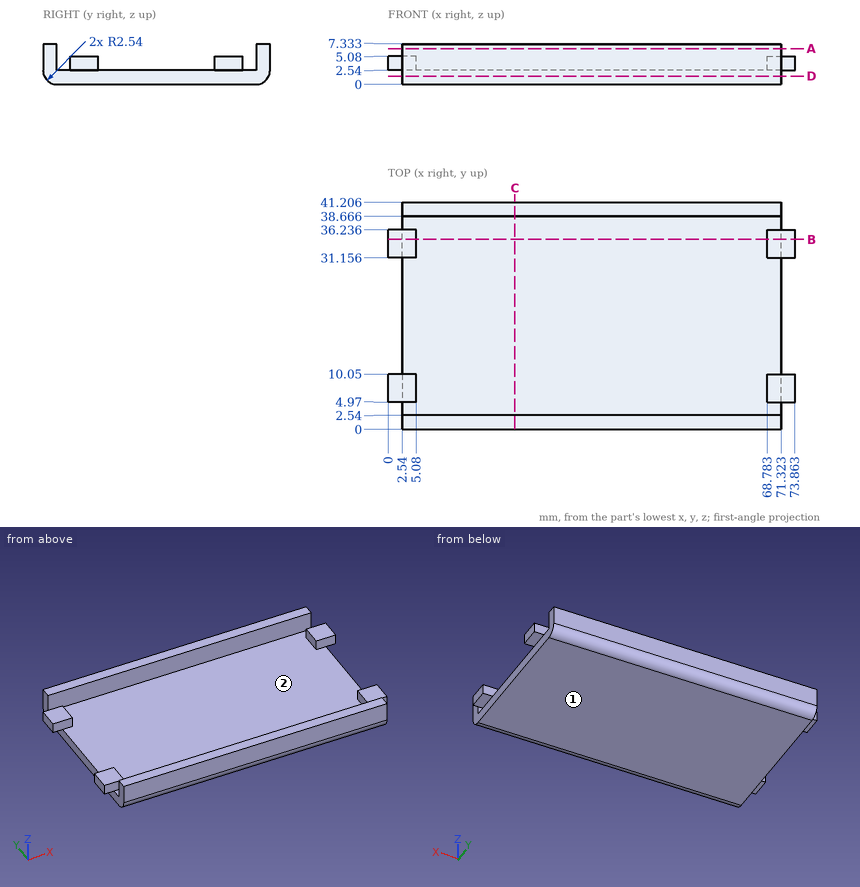
Answer from the drawing. Dimensions are ordinates in mm from the lowest x, y and z of the part. Give positions to 0.01 mm unless a question says otherwise; leave off trailing zeros. Write each loop counter-clockwise with the first axis right and the second up, starting at its lowest first coordinate (ties: lowest second). Pieces come first, ordered by that corner, then holes.
1) Find the intervals of material crossed by L1, parallel to X at y = 9, z = 2.75; L2, parallel to Y at x = 61, z = 6.75; L3, parallel to X at y = 16, z = 0.5, in increasing order.
2) Section C-C (x = 23) is taken. Write down the section's boundary in (y, z), and give its area (3 significant figures).
3) Section A-A (z = 6.5) is taken. Write down the section's boundary in (x, y).
4) For a pull along X with two mould halves and no side action, classify the marked faces 1 and 2 as pulls with the +X half, pulls with the -X half, needs draft (parallel to the pull), parting line crosses it, or undercut.
5) Given P1, Ø2, axis at y = 17, z = 4.5, coming from the +X side; P2, Ø1.3, axis at y = 34, z = 4, coming from the -X side; P3, Ø5.5, axis at x = 3, y = 34, coming from the +Z side; P4, Ø0.8, axis at x = 1.5, z = 4, coming from the +Y side, each flat-ended and moving along its own axis, determine where each tip first touches the part or whether it passes through.
6) Section B-B (y = 34.5) is taken. Write down the section's boundary in (x, z).
7) Section D-D (z = 1.5) is taken. Write down the section's boundary in (x, y).
Response:
1. L1: x = 0 to 5.08, 68.78 to 73.86
1. L2: y = 0 to 2.54, 38.67 to 41.21
1. L3: x = 2.54 to 71.32
2. outline: (0, 2.54) arc R2.54 ccw to (2.54, 0) - (38.67, 0) arc R2.54 ccw to (41.21, 2.54) - (41.21, 7.33) - (38.67, 7.33) - (38.67, 2.54) - (2.54, 2.54) - (2.54, 7.33) - (0, 7.33) - close
2. area: 126 mm2
3. outline: (2.54, 0) - (71.32, 0) - (71.32, 2.54) - (2.54, 2.54) - close; (2.54, 38.67) - (71.32, 38.67) - (71.32, 41.21) - (2.54, 41.21) - close
4. face 1: needs draft
4. face 2: undercut
5. P1: passes through
5. P2: stops at x = 0
5. P3: stops at z = 5.08
5. P4: stops at y = 36.24
6. outline: (0, 2.54) - (2.54, 2.54) - (2.54, 0) - (71.32, 0) - (71.32, 2.54) - (73.86, 2.54) - (73.86, 5.08) - (68.78, 5.08) - (68.78, 2.54) - (5.08, 2.54) - (5.08, 5.08) - (0, 5.08) - close
7. outline: (2.54, 0.22) - (71.32, 0.22) - (71.32, 40.98) - (2.54, 40.98) - close
